Work out the finished part from the listing and answer in its coordinate system (mm). A direction names the side the tool comes from. Round coordinates to 2 decimals unless told otherwise and drop trailing zeros. Write each loop counter-clockwise with the first axis right and the second up, starting at its lowest first coordinate (ties: lowest second). Pieces come first, ordered by that corner, then holes. Notation, with made-up numbers: (42, -6) -> (76, -6) arc R20 ccw to (76, 13) -> close; hole circle Ø11 at (59, -18). An arc over 180 degrees is marked (long way). Answer as a JSON object with one key per item and string values. Group by question number.
from build123d import *

# Parameters (mm, degrees)
SKETCH_R     = 1.6
PAD_DEPTH    = 3
SKETCH001_W  = 6.4
SKETCH001_H  = 89.324535
POCKET_DEPTH = 1


with BuildPart() as part:
    # Sketch → Pad (new body)
    with BuildSketch(Plane.XY):
        Polygon((18, 0), (18, 61), (38.4, 61), (38.400002, 0), align=None)
        with Locations((21.5, 54)):
            Circle(SKETCH_R, mode=Mode.SUBTRACT)
        with Locations((21.5, 7)):
            Circle(SKETCH_R, mode=Mode.SUBTRACT)
        with Locations((34.9, 7)):
            Circle(SKETCH_R, mode=Mode.SUBTRACT)
        with Locations((34.900002, 54)):
            Circle(SKETCH_R, mode=Mode.SUBTRACT)
        with Locations((34.9, 30.5)):
            Circle(SKETCH_R, mode=Mode.SUBTRACT)
        with Locations((21.5, 30.5)):
            Circle(SKETCH_R, mode=Mode.SUBTRACT)
    extrude(amount=PAD_DEPTH)

    # Sketch001 (on Face12 of Pad) → Pocket (cut)
    with BuildSketch(Plane.XY.offset(3)):
        with Locations((28.2, 34.865138)):
            Rectangle(SKETCH001_W, SKETCH001_H)
    extrude(amount=-POCKET_DEPTH, mode=Mode.SUBTRACT)


solid = part.part
1) A cutting plane is placed at B-B on x = 21.5. Determine the outline of the cut face in (y, z), plus the area to 3 significant figures.
2) Straight lines are drawn through the part: L1, parallel to Y at x = 21.5, z = 0.7; L2, parallel to X at y = 50.5, z = 2.5; L3, parallel to X at y = 8, z = 1.1. For each, find the intervals that lie inside material, in ascending order.
3) A cutting plane is placed at C-C on z = 1.2. Determine the outline of the cut face in (x, y).
4) A cutting plane is placed at A-A on y = 7. Determine the outline of the cut face in (x, z).
5) A tool of negligible diameter and unlimited length cuts with its end or side. For faces 1 (the face through (31.4, 30.1, 2.5)), 2 (the face through (33.3, 54.07, 1.48)), from which of +Z, -Z, +X, -X, +Y, -Y can it reach the whole face along a straight path? Write none if from no direction.
6) This flat-tipped pin is pushed along its axis until it touches: P1, Ø1.9, axis at x = 29, y = 25, coming from the +Z side. Where does it stop, or does it pass through?
7) For a pull along Y with two mould halves and no side action, classify faces 3 (the face through (36.426, 30.981, 1.479)), 4 (the face through (28, 31, 0)), 5 (the face through (28, 0, 1)) as released by +Y, released by -Y, zero draft, split by the parting line, or undercut.
8) A cutting plane is placed at D-D on y = 42.5. Determine the outline of the cut face in (x, z).
Established:
{
 "1": {"outline": "(0, 0) -> (5.4, 0) -> (5.4, 3) -> (0, 3) -> close; (8.6, 0) -> (28.9, 0) -> (28.9, 3) -> (8.6, 3) -> close; (32.1, 0) -> (52.4, 0) -> (52.4, 3) -> (32.1, 3) -> close; (55.6, 0) -> (61, 0) -> (61, 3) -> (55.6, 3) -> close", "area": "154 mm²"},
 "2": {"L1": "y = 0 to 5.4, 8.6 to 28.9, 32.1 to 52.4, 55.6 to 61", "L2": "x = 18 to 25, 31.4 to 38.4", "L3": "x = 18 to 20.25, 22.75 to 33.65, 36.15 to 38.4"},
 "3": {"outline": "(18, 0) -> (38.4, 0) -> (38.4, 61) -> (18, 61) -> close; hole circle Ø3.2 at (21.5, 7); hole circle Ø3.2 at (21.5, 30.5); hole circle Ø3.2 at (21.5, 54); hole circle Ø3.2 at (34.9, 7); hole circle Ø3.2 at (34.9, 30.5); hole circle Ø3.2 at (34.9, 54)"},
 "4": {"outline": "(18, 0) -> (19.9, 0) -> (19.9, 3) -> (18, 3) -> close; (23.1, 0) -> (33.3, 0) -> (33.3, 3) -> (31.4, 3) -> (31.4, 2) -> (25, 2) -> (25, 3) -> (23.1, 3) -> close; (36.5, 0) -> (38.4, 0) -> (38.4, 3) -> (36.5, 3) -> close"},
 "5": {"face 1": "+Z, +Y, -Y", "face 2": "+Z, -Z"},
 "6": {"P1": "stops at z = 2"},
 "7": {"face 3": "undercut", "face 4": "zero draft", "face 5": "released by -Y"},
 "8": {"outline": "(18, 0) -> (38.4, 0) -> (38.4, 3) -> (31.4, 3) -> (31.4, 2) -> (25, 2) -> (25, 3) -> (18, 3) -> close"}
}
